Answer from the drawing. Dimensions are ordinates in mm from the lowest x, y and z of the part. A direction names the side the tool comes from. Round coordinates to 2 decimals unless told otherwise and drop trailing zeros. Write each loop counter-clockwise with the first axis right and the second up, starting at its lowest first coordinate (ties: lowest second). Pieces come first, ordered by that corner, then holes. Notation, with made-up numbers: (83.25, 68.5) - (133.25, 68.5) arc R13 ccw to (133.25, 76.5) - close; hole circle Ø7 at (27, 78). An arc over 180 degrees is marked (long way). Answer as a JSON object with one key per item and string values.
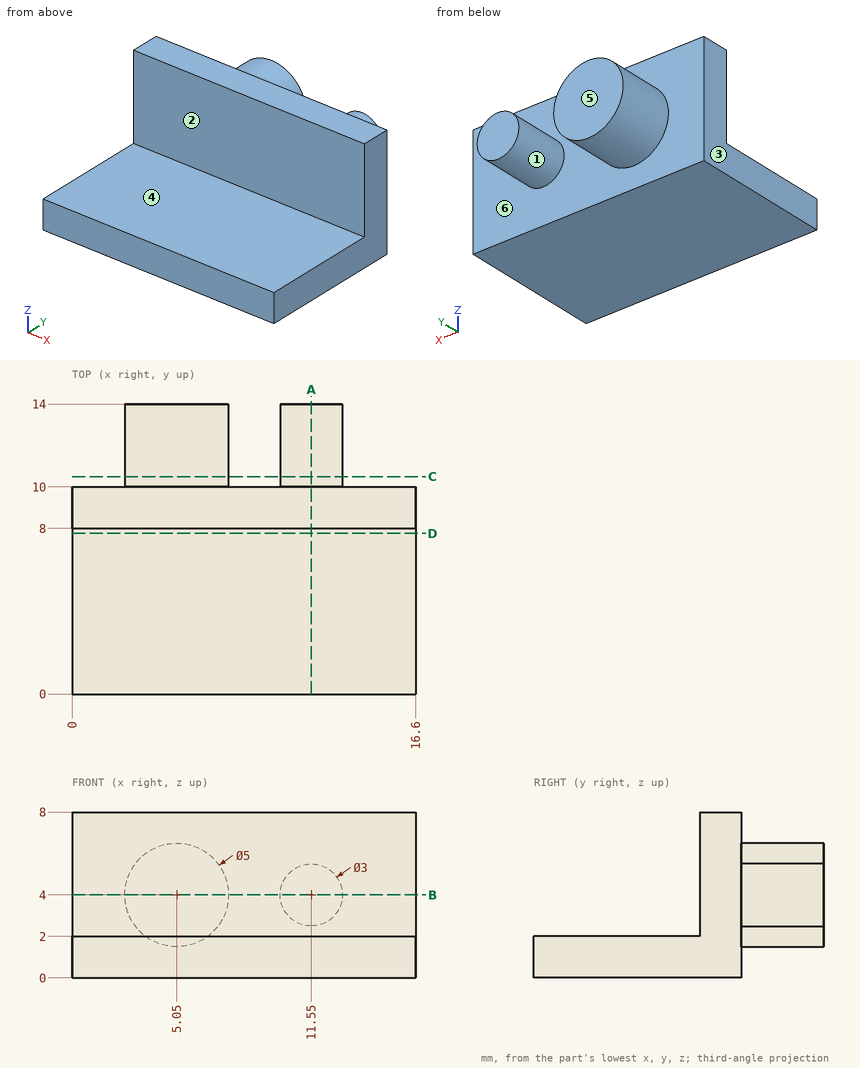
Item 1: Each of these flat-tipped pins is pushed along its axis until it touches: P1, Ø3, axis at x = 5, y = 10.5, coming from the +Z side; P2, Ø2, axis at x = 6, y = 6, coming from the +Z side; P3, Ø3, axis at x = 6.5, z = 5, coming from the -Y side. Where does it stop, or does it pass through?
Results found:
{"P1": "z = 8", "P2": "z = 2", "P3": "y = 8"}
Item 2: A cutting plane is placed at C-C (y = 10.5). Write down the section's boundary in (x, z), and give its area (3 significant figures).
Results found:
{"outline": "circle Ø5 at (5.05, 4); circle Ø3 at (11.55, 4)", "area": "26.7 mm²"}
Item 3: A cutting plane is placed at A-A (x = 11.55). Write down the section's boundary in (y, z), and give its area (3 significant figures).
Results found:
{"outline": "(0, 0) - (10, 0) - (10, 2.5) - (14, 2.5) - (14, 5.5) - (10, 5.5) - (10, 8) - (8, 8) - (8, 2) - (0, 2) - close", "area": "44.0 mm²"}
Item 4: Consider line 1 along X through (y, z) = (13.25, 4); line 2 along Z through (x, y) = (11, 6); line 3 along Y through (x, z) = (7.25, 4.75). Determine where each line is inside the solid, lowest interval first.
Results found:
{"line 1": "2.55 to 7.55, 10.05 to 13.05", "line 2": "0 to 2", "line 3": "8 to 14"}
Item 5: A cutting plane is placed at B-B (z = 4). Write down the section's boundary in (x, y).
Results found:
{"outline": "(0, 8) - (16.6, 8) - (16.6, 10) - (13.05, 10) - (13.05, 14) - (10.05, 14) - (10.05, 10) - (7.55, 10) - (7.55, 14) - (2.55, 14) - (2.55, 10) - (0, 10) - close"}
Item 6: For the marked faces 4, 5 and 6, determine the directions among +Z, -Z, +X, -X, +Y, -Y from which every point of the face is accessible in a straight line to the end or side of a thin tool.
Results found:
{"face 4": "+Z, +X, -X, -Y", "face 5": "+Z, -Z, +X, -X, +Y", "face 6": "+Y"}
Item 7: A cutting plane is placed at D-D (y = 7.75). Write down the section's boundary in (x, z), and give its area (3 significant figures).
Results found:
{"outline": "(0, 0) - (16.6, 0) - (16.6, 2) - (0, 2) - close", "area": "33.2 mm²"}
Item 8: Determine the mould class of the marked faces 1, 2 and 3 for opening direction X: pulls with the +X half, pulls with the -X half, needs draft (parallel to the pull), parting line crosses it, or undercut.
Results found:
{"face 1": "undercut", "face 2": "needs draft", "face 3": "pulls with the -X half"}
